Geometry check sheet. Reference: drawing and pictorial views, mm from the part's lowest x, y, z. Coordinates: 2 decimals unless noted, no trailing zeros. Order: outer loops, then holes, each group sorted by start corner. A loop starts at its lowest first (then second) coordinate and runs counter-clockwise, first axis right, second up. Notation, with made-up numbers: M 88,-27 L 98,-27 A17 ccw 98,-3 Z; hole C 81.5,-40 d6. An arc over 180 degrees is marked long. Return JSON: item names as keys, results as strings.
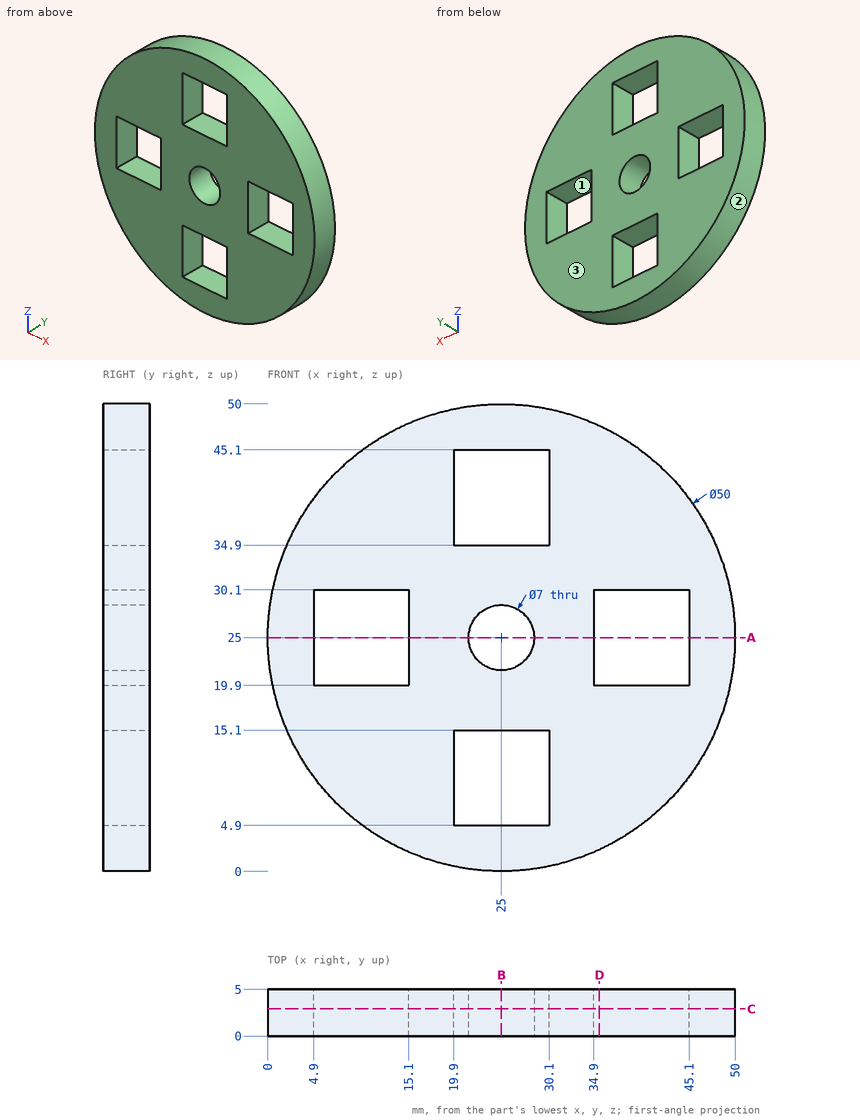
Q1. Cross-section at D-D, the plane x = 35.5. Record the boundary of the cut face in (y, z).
Values:
{"outline": "M 0,2.31 L 5,2.31 L 5,19.9 L 0,19.9 Z; M 0,30.1 L 5,30.1 L 5,47.69 L 0,47.69 Z"}
Q2. Cross-section at B-B, the plane x = 25. Record the boundary of the cut face in (y, z), and give its area (3 significant figures).
Values:
{"outline": "M 0,0 L 5,0 L 5,4.9 L 0,4.9 Z; M 0,15.1 L 5,15.1 L 5,21.5 L 0,21.5 Z; M 0,28.5 L 5,28.5 L 5,34.9 L 0,34.9 Z; M 0,45.1 L 5,45.1 L 5,50 L 0,50 Z", "area": "113 mm^2"}
Q3. Draft check along X on the marked faces 1, 2 and 3. Enter one of: pulls with the +X half, pulls with the -X half, needs draft (parallel to the pull), parting line crosses it, or undercut.
Values:
{"face 1": "undercut", "face 2": "parting line crosses it", "face 3": "needs draft"}
Q4. Cross-section at C-C, the plane y = 2.9. Record the boundary of the cut face in (x, z).
Values:
{"outline": "C 25,25 d50; hole M 4.9,19.9 L 15.1,19.9 L 15.1,30.1 L 4.9,30.1 Z; hole M 19.9,4.9 L 30.1,4.9 L 30.1,15.1 L 19.9,15.1 Z; hole M 19.9,34.9 L 30.1,34.9 L 30.1,45.1 L 19.9,45.1 Z; hole C 25,25 d7; hole M 34.9,19.9 L 45.1,19.9 L 45.1,30.1 L 34.9,30.1 Z"}
Q5. Cross-section at A-A, the plane z = 25. Record the boundary of the cut face in (x, y), and give its area (3 significant figures).
Values:
{"outline": "M 0,0 L 4.9,0 L 4.9,5 L 0,5 Z; M 15.1,0 L 21.5,0 L 21.5,5 L 15.1,5 Z; M 28.5,0 L 34.9,0 L 34.9,5 L 28.5,5 Z; M 45.1,0 L 50,0 L 50,5 L 45.1,5 Z", "area": "113 mm^2"}
Q6. Go/stop test with flat-tipped pins: pin 1 (2.5 mm diameter, centred on y = 2.5, z = 9.5, fed in from -X); pin 2 (1 mm diameter, centred on x = 10.5, y = 0.5, fed in from -Z); pin 3 (2.5 mm diameter, centred on y = 2.5, z = 23.5, fed in from -X); pin 4 (3 mm diameter, centred on x = 34, z = 5.5, fed in from -Y). Record where each tip stops, or that it passes through.
Values:
{"pin 1": "x = 4.46", "pin 2": "z = 4.29", "pin 3": "x = 0", "pin 4": "y = 0"}
Q7. Material ranges on line 1 along X through (y, z) = (3.95, 25); line 2 along X through (y, z) = (2.9, 20.5), recorded low to high.
Values:
{"line 1": "0 to 4.9, 15.1 to 21.5, 28.5 to 34.9, 45.1 to 50", "line 2": "0.41 to 4.9, 15.1 to 34.9, 45.1 to 49.59"}
